Could you check a few things on this model? Use its own coordinates, in mm. Face numbers are marked on the shaded views. Coordinates: 2 decimals unless noted, no trailing zeros. Loops run counter-clockwise (first coordinate to the right, second up) from the corner with the lowest first, then second, coordinate; pieces in that order, holes last.
1) Will these pins go through, and if not, where does the flat tip stop? P1, Ø3, axis at x = -15, y = -7.5, coming from the -Z side; P2, Ø10, axis at x = -2.5, y = 0, coming from the -Z side.
2) If I drill on line 1 along X through (y, z) = (-11, 5); line 2 along Z through (x, y) = (0, 1.5); line 3 along Z through (x, y) = (19.5, -15.5), over which ranges is the centre line in solid material (lowest first)?
3) Imagine slicing it at B-B on x = -15. Please give me the cut outline in (y, z), plus the area to 3 significant figures.
4) Imagine slicing it at A-A on y = 4.5. Please give me the cut outline in (x, z).
5) Imagine slicing it at C-C on x = 10. Please give me the cut outline in (y, z), plus the area to 3 significant figures.
6) Thinking about a two-plate mould opening in X: for the marked faces 1, 2 and 3, which applies, released by +X, released by -X, zero draft, split by the parting line, or undercut?
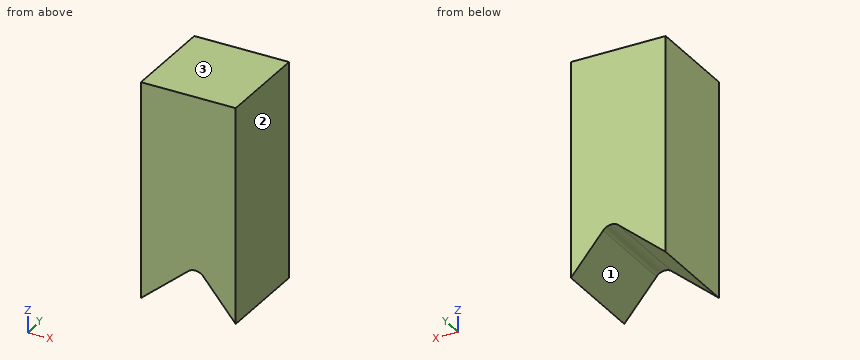
```python
from build123d import *

# Parameters (mm, degrees)
F0_W     = 44
F0_H     = 44
F1_DEPTH = 100
F3_DEPTH = 44.001
F4_R     = 5


with BuildPart() as f1:
    # F0 (on Top) → F1 (new body)
    with BuildSketch(Plane.XY):
        Rectangle(F0_W, F0_H)
    extrude(amount=F1_DEPTH)

    # F2 (on face) → F3 (cut, through all)
    with BuildSketch(Plane.XZ.offset(22)):
        Polygon((3.82026, 21.665771), (-22, 0), (22, 0), align=None)
    extrude(amount=-F3_DEPTH, mode=Mode.SUBTRACT)

    # F4
    f4_edges = [f1.edges().sort_by_distance(p)[0] for p in [
        (3.82026, 0, 21.665771),
    ]]
    fillet(f4_edges, radius=F4_R)


solid = f1.part
```
Filled in:
1. P1: stops at z = 4.62
1. P2: stops at z = 12.17
2. line 1: x = -22 to -16.04, 17.8 to 22
2. line 2: z = 18.46 to 100
2. line 3: z = 2.98 to 100
3. outline: (-22, 5.87) - (22, 5.87) - (22, 100) - (-22, 100) - close
3. area: 4,140 mm2
4. outline: (-22, 0) - (-0.01, 18.45) arc R5 cw to (7.03, 17.84) - (22, 0) - (22, 100) - (-22, 100) - close
5. outline: (-22, 14.3) - (22, 14.3) - (22, 100) - (-22, 100) - close
5. area: 3,770 mm2
6. face 1: undercut
6. face 2: released by +X
6. face 3: zero draft
